Work out the finished part from the listing and answer in its coordinate system (mm). A direction names the side the tool comes from. Give positions to 0.01 mm unless a question says otherwise; leave off trailing zeros. Loops run counter-clockwise (first coordinate to the right, second up) from the corner with the lowest first, then second, coordinate; pieces in that order, holes last. Notation, with made-up numbers: (-2, 25.5) - (7, 25.5) arc R8 cw to (7, 32.5) - close; hole circle Ø8 at (33.5, -23.75). An arc over 180 degrees is marked (long way). One line per item, written item: value.
from build123d import *

# Parameters (mm, degrees)
SKETCH1_W               = 77
SKETCH1_H               = 12
BOSS_EXTRUDE1_DEPTH     = 10
SKETCH2_R               = 1.25
CUT_EXTRUDE1_DEPTH      = 12
BOSS_EXTRUDE2_OUTLINE_W = 77
BOSS_EXTRUDE2_OUTLINE_H = 20
BOSS_EXTRUDE2_DEPTH     = 5
SKETCH4_W               = 77
SKETCH4_H               = 22
BOSS_EXTRUDE3_DEPTH     = 5
SKETCH5_R               = 1.25
CUT_EXTRUDE2_DEPTH      = 12
SKETCH7_W               = 77
SKETCH7_H               = 22
BOSS_EXTRUDE4_DEPTH     = 15
SKETCH8_R               = 1.5
CUT_EXTRUDE3_DEPTH      = 83.540898953


# Read off the part's stored shape, not the designer's step: Boss-Extrude2
with BuildPart() as part:
    # Sketch1 → Boss-Extrude1 (new body)
    with BuildSketch(Plane.XY):
        with Locations((38.5, 6)):
            Rectangle(SKETCH1_W, SKETCH1_H)
    extrude(amount=BOSS_EXTRUDE1_DEPTH)

    # Sketch2 → Cut-Extrude1 (cut)
    with BuildSketch(Plane(origin=(77, 0, 0), x_dir=(0, 0, -1), z_dir=(1, 0, 0))):
        with Locations((-5, 3)):
            Circle(SKETCH2_R)
        with Locations((-5, 9)):
            Circle(SKETCH2_R)
    extrude(amount=-CUT_EXTRUDE1_DEPTH, mode=Mode.SUBTRACT)

    # Boss-Extrude2 outline → Boss-Extrude2 (add)
    with BuildSketch(Plane(origin=(0, 12, 0), x_dir=(1, 0, 0), z_dir=(0, 1, 0))):
        with Locations((38.5, -10)):
            Rectangle(BOSS_EXTRUDE2_OUTLINE_W, BOSS_EXTRUDE2_OUTLINE_H)
    boss_extrude2 = extrude(amount=BOSS_EXTRUDE2_DEPTH)

    # Mirror2: Boss-Extrude2 across plane
    add(boss_extrude2.mirror(Plane(origin=(0, 6, 0), x_dir=(0, 0, 1), z_dir=(0, -1, 0))))

    # Sketch4 → Boss-Extrude3 (add)
    with BuildSketch(Plane(origin=(0, 0, 0), x_dir=(-1, 0, 0), z_dir=(0, 0, -1))):
        with Locations((-38.5, 6)):
            Rectangle(SKETCH4_W, SKETCH4_H)
    extrude(amount=BOSS_EXTRUDE3_DEPTH)

    # Sketch5 → Cut-Extrude2 (cut)
    with BuildSketch(Plane.ZY):
        with Locations((6, 6)):
            Circle(SKETCH5_R)
    extrude(amount=-CUT_EXTRUDE2_DEPTH, mode=Mode.SUBTRACT)

    # Sketch7 → Boss-Extrude4 (add)
    with BuildSketch(Plane(origin=(0, 0, -5), x_dir=(-1, 0, 0), z_dir=(0, 0, -1))):
        with Locations((-38.5, 6)):
            Rectangle(SKETCH7_W, SKETCH7_H)
    extrude(amount=BOSS_EXTRUDE4_DEPTH)

    # Sketch8 → Cut-Extrude3 (cut, through all)
    with BuildSketch(Plane.XZ.offset(5)):
        with Locations((19.25, -12.5)):
            Circle(SKETCH8_R)
        with Locations((38.5, -12.5)):
            Circle(SKETCH8_R)
        with Locations((57.75, -12.5)):
            Circle(SKETCH8_R)
    extrude(amount=-CUT_EXTRUDE3_DEPTH, mode=Mode.SUBTRACT)


solid = part.part
1. Find the intervals of material crossed by line 1 along Y through (x, z) = (74, 5); line 2 along Z through (x, y) = (38.5, 8.25); line 3 along Y through (x, z) = (60, 15), in increasing order.
Output:
line 1: y = -5 to 1.75, 4.25 to 7.75, 10.25 to 17
line 2: z = -20 to -14, -11 to 10
line 3: y = -5 to 0, 12 to 17
2. Flat-ended cylindrical pins translate along their axes: pin 1 Ø0.8 at (y, z) = (5.5, 5.5) entering from -X; pin 2 Ø6 at (x, y) = (20.5, 6.5) entering from +Z; pin 3 Ø2 at (y, z) = (9, 5) entering from -X; pin 4 Ø0.8 at (y, z) = (9.5, 5) entering from +X. Find the tip coordinate at first contact, or state that the pin passes through.
Output:
pin 1: stops at x = 12
pin 2: stops at z = 10
pin 3: stops at x = 0
pin 4: stops at x = 65
3. Section B-B (x = 38.5) is taken. Write down the section's boundary in (y, z).
Output:
outline: (-5, -20) - (17, -20) - (17, -14) - (-5, -14) - close; (-5, -11) - (17, -11) - (17, 20) - (12, 20) - (12, 10) - (0, 10) - (0, 20) - (-5, 20) - close
4. Section C-C (y = 3) is taken. Write down the section's boundary in (x, z), and give its area (3 significant figures).
Output:
outline: (0, -20) - (77, -20) - (77, 3.75) - (65, 3.75) - (65, 6.25) - (77, 6.25) - (77, 10) - (0, 10) - close; hole circle Ø3 at (19.25, -12.5); hole circle Ø3 at (38.5, -12.5); hole circle Ø3 at (57.75, -12.5)
area: 2,260 mm²
5. For faces 4 (the cylindrical face through (71.084, 3.845, 5.921)), 5 (the flat face through (38, -2, 20)), 6 (the cylindrical face through (5.92, 4.78, 5.73)), 7 (the flat face through (39, 6, -20)), 8 (the flat face through (38, 12, 15)), determine the directions among +Z, -Z, +X, -X, +Y, -Y from which every point of the face is accessible in a straight line to the end or side of a thin tool.
Output:
face 4: +X
face 5: +Z, +X, -X, +Y, -Y
face 6: -X
face 7: -Z, +X, -X, +Y, -Y
face 8: +Z, +X, -X
6. Section D-D (z = -12.5) is taken. Write down the section's boundary in (x, y).
Output:
outline: (0, -5) - (17.75, -5) - (17.75, 17) - (0, 17) - close; (20.75, -5) - (37, -5) - (37, 17) - (20.75, 17) - close; (40, -5) - (56.25, -5) - (56.25, 17) - (40, 17) - close; (59.25, -5) - (77, -5) - (77, 17) - (59.25, 17) - close
7. The mould has two halves that part along Y. Classify faces 1 (the flat face through (39, 17, 0)), 2 (the flat face through (0, 6, 0)), 3 (the flat face through (12, 6, 6)): released by +Y, released by -Y, zero draft, split by the parting line, or undercut.
Output:
face 1: released by +Y
face 2: zero draft
face 3: undercut
8. Section A-A (z = 16.5) is taken. Write down the section's boundary in (x, y).
Output:
outline: (0, -5) - (77, -5) - (77, 0) - (0, 0) - close; (0, 12) - (77, 12) - (77, 17) - (0, 17) - close
